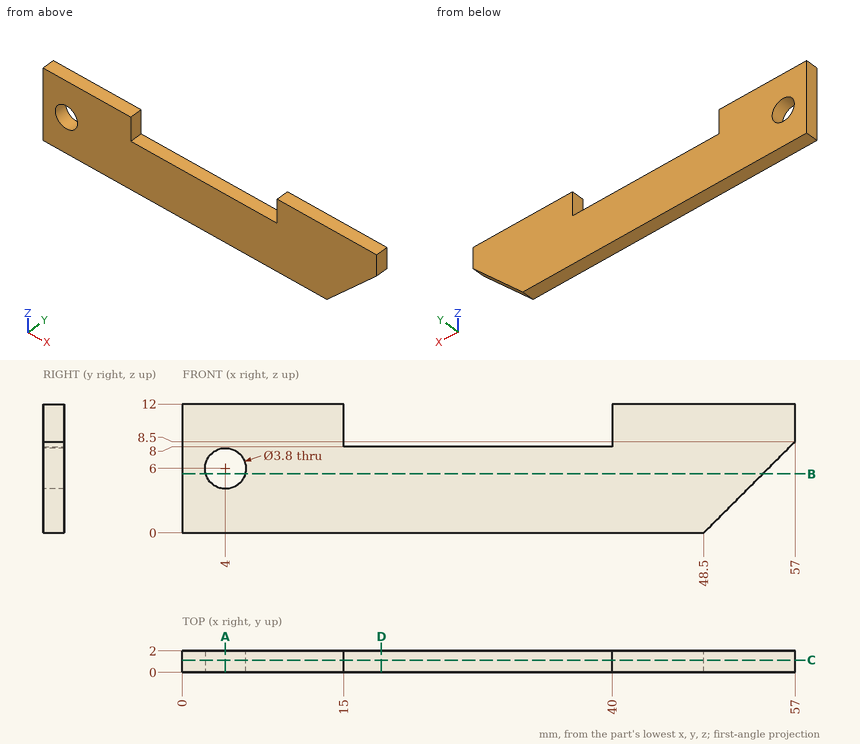
For this review, use the dimensioned drawing (mm, ordinates from the lowest corner) and the shaded views. Give positions to 0.01 mm unless a question says otherwise; leave off trailing zeros. Order: outer loops, then holes, each group sorted by start corner. A loop starts at its lowest first (then second) coordinate and runs counter-clockwise, first axis right, second up.
1) Take a section at A-A (x = 4). Give the boundary of the cut face in (y, z).
2) Wall thickness on line 1 (Z direction, x = 4, y = 1.55); line 2 (X direction, y = 0.25, z = 9.5); line 3 (Z direction, x = 24, y = 0.95): over which ranges is each line inside the solid? List them lowest first.
3) Take a section at B-B (z = 5.5). Give the boundary of the cut face in (x, y), then the cut area to 3 significant figures.
4) Take a section at C-C (y = 1.15). Give the boundary of the cut face in (x, z), then the cut area to 3 significant figures.
5) Take a section at D-D (x = 18.5). Give the boundary of the cut face in (y, z), then the cut area to 3 significant figures.
Derived:
1. outline: (0, 0) - (2, 0) - (2, 4.1) - (0, 4.1) - close; (0, 7.9) - (2, 7.9) - (2, 12) - (0, 12) - close
2. line 1: z = 0 to 4.1, 7.9 to 12
2. line 2: x = 0 to 15, 40 to 57
2. line 3: z = 0 to 8
3. outline: (0, 0) - (2.17, 0) - (2.17, 2) - (0, 2) - close; (5.83, 0) - (54, 0) - (54, 2) - (5.83, 2) - close
3. area: 101 mm2
4. outline: (0, 0) - (48.5, 0) - (57, 8.5) - (57, 12) - (40, 12) - (40, 8) - (15, 8) - (15, 12) - (0, 12) - close; hole circle Ø3.8 at (4, 6)
4. area: 537 mm2
5. outline: (0, 0) - (2, 0) - (2, 8) - (0, 8) - close
5. area: 16.0 mm2
